```python
from build123d import *

# Parameters (mm, degrees)
BOSS_EXTRUDE1_DEPTH = 17.5
M20_TAPPED_HOLE1_D  = 17.5


with BuildPart() as part:
    # Sketch1 → Boss-Extrude1 (new, symmetric)
    with BuildSketch(Plane(origin=(0, 0, 0), x_dir=(1, 0, 0), z_dir=(0, 1, 0))):
        Polygon((-10.8, 0), (-17.45, 0), (-17.45, 11.5), (-14.95, 14), (14.95, 14), (17.45, 11.5), (17.45, 0), (10.8, 0), (10.8, -14), (-10.8, -14), align=None)
    extrude(amount=BOSS_EXTRUDE1_DEPTH, both=True)

    # M20 Tapped Hole1 (through all)
    with Locations(Plane.XY.offset(14)):
        with Locations((0, 0)):
            Hole(M20_TAPPED_HOLE1_D / 2)


solid = part.part
```
Geometry check sheet. Reference: the model listing, model coordinates, mm. A direction names the side the tool comes from. Coordinates: 2 decimals unless noted, no trailing zeros. Order: outer loops, then holes, each group sorted by start corner. A loop starts at its lowest first (then second) coordinate and runs counter-clockwise, first axis right, second up. Notation, with made-up numbers: M -35.75,28.25 L -5.75,28.25 A22 cw -5.75,56.25 Z; hole C 46,33 d3. An arc over 180 degrees is marked long. One line per question, with ' | ' between items. Start each with the question number.
Item 1: Set-up check for faces 1 (the flat face through (-10.8, 0, 7)), 2 (the flat face through (-16.22, 0.25, -12.73)), 3 (the flat face through (14, 0, 0)): record each of +Z, -Z, +X, -X, +Y, -Y from which the full face is reachable in a straight line by a thin tool's end or side.
Item 2: Cross-section at D-D on y = 14.5. Enter the section's corners in (x, z).
Item 3: Draft check along Y on faces 4 (the flat face through (-17.45, 0, -6)), 5 (the cylindrical face through (6.944, -5.324, -0.196)), 6 (the flat face through (0, 17.5, -3)), 7 (the flat face through (0, -17.5, -3)). Enter one of: pulls with the +Y half, pulls with the -Y half, needs draft (parallel to the pull), parting line crosses it, or undercut.
Item 4: Cross-section at B-B on y = 0. Enter the section's corners in (x, z), then the cut area to 3 significant figures.
Item 5: Cross-section at A-A on x = 0. Enter the section's corners in (y, z), then the cut area to 3 significant figures.
Item 6: Material ranges on L1, parallel to Y at x = 0, z = 7; L2, parallel to Z at x = 12, y = -4.5; L3, parallel to Y at x = -4.5, z = -8.75, recorded low to high. Write a range as [from, to].
Item 7: Cross-section at C-C on z = -1. Enter the section's corners in (x, y).
Item 8: Gauge pin test, flat ends, axial feed: pin 1 (2 mm diameter, centred on x = -13, y = 4, fed in from +Z); pin 2 (10 mm diameter, centred on y = 10, z = 6, fed in from +X); pin 3 (8 mm diameter, centred on y = -3, z = 8, fed in from -X); pin 4 (6 mm diameter, centred on y = 9, z = 1.5, fed in from +X). Record the tip position at first contact, or that the pin passes through.
Findings:
1) face 1: +Z, -X, +Y, -Y | face 2: -Z, -X, +Y, -Y | face 3: +Z, +X, +Y, -Y
2) outline: M -17.45,-11.5 L -14.95,-14 L 14.95,-14 L 17.45,-11.5 L 17.45,0 L 10.8,0 L 10.8,14 L -10.8,14 L -10.8,0 L -17.45,0 Z
3) face 4: needs draft | face 5: undercut | face 6: pulls with the +Y half | face 7: pulls with the -Y half
4) outline: M -17.45,-11.5 L -14.95,-14 L -8.75,-14 L -8.75,14 L -10.8,14 L -10.8,0 L -17.45,0 Z; M 8.75,-14 L 14.95,-14 L 17.45,-11.5 L 17.45,0 L 10.8,0 L 10.8,14 L 8.75,14 Z | area: 295 mm²
5) outline: M -17.5,-14 L -8.75,-14 L -8.75,14 L -17.5,14 Z; M 8.75,-14 L 17.5,-14 L 17.5,14 L 8.75,14 Z | area: 490 mm²
6) L1: y = [-17.5, -8.75], [8.75, 17.5] | L2: z = [-14, 0] | L3: y = [-17.5, -7.5], [7.5, 17.5]
7) outline: M -17.45,-17.5 L 17.45,-17.5 L 17.45,17.5 L -17.45,17.5 Z; hole C 0,0 d17.5
8) pin 1: stops at z = 0 | pin 2: stops at x = 10.8 | pin 3: stops at x = -10.8 | pin 4: stops at x = 17.45
